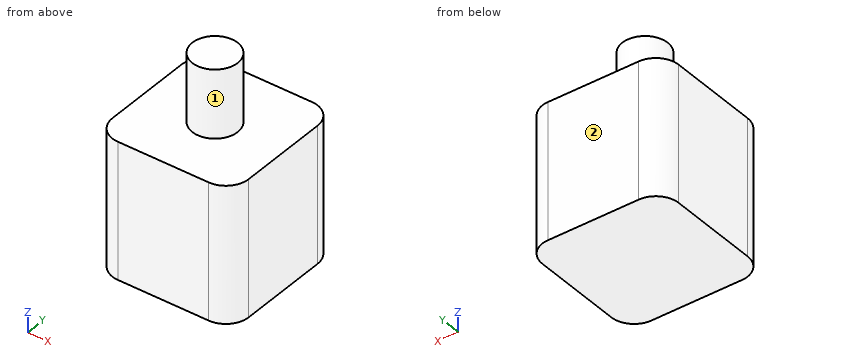
from build123d import *

# Parameters (mm, degrees)
SKETCH1_W           = 60
SKETCH1_H           = 60
BOSS_EXTRUDE1_DEPTH = 30
SKETCH2_R           = 10
BOSS_EXTRUDE2_DEPTH = 30
FILLET1_R           = 10


with BuildPart() as part:
    # Sketch1 → Boss-Extrude1 (new body, symmetric)
    with BuildSketch(Plane.XY):
        Rectangle(SKETCH1_W, SKETCH1_H)
    extrude(amount=BOSS_EXTRUDE1_DEPTH, both=True)

    # Sketch2 → Boss-Extrude2 (add)
    with BuildSketch(Plane.XY.offset(30)):
        Circle(SKETCH2_R)
    extrude(amount=BOSS_EXTRUDE2_DEPTH)

    # Fillet1
    fillet1_edges = [part.edges().sort_by_distance(p)[0] for p in [
        (30, -30, 0),
        (-30, -30, 0),
        (-30, 30, 0),
        (30, 30, 0),
    ]]
    fillet(fillet1_edges, radius=FILLET1_R)


solid = part.part
Work out the finished part from the listing and answer in its coordinate system (mm). Face numbers are marked on the shaded views. A direction names the side the tool comes from. Round coordinates to 2 decimals unless told otherwise and drop trailing zeros. Loops run counter-clockwise (first coordinate to the right, second up) from the corner with the lowest first, then second, coordinate; pieces in that order, holes last. Notation, with made-up numbers: (39.25, 36) - (59.25, 36) arc R13 cw to (59.25, 51) - close; hole circle Ø6 at (-11.75, -3). An arc over 180 degrees is marked (long way). Use one line per item in the form item = value. Start each with the question number.
(1) Find section C-C on z = 45. Determine the outline of the cut face in (x, y).
(2) Which of the six approach directions +Z, -Z, +X, -X, +Y, -Y give full straight-line access (tool end or side, diameter ignored) to the marked faces 1 and 2?
(3) Find section A-A on y = 0. Determine the outline of the cut face in (x, z), and give its area (3 significant figures).
(4) Find section D-D on y = -18. Determine the outline of the cut face in (x, z), and give its area (3 significant figures).
(5) Consider line 1 (Z direction, x = -25, y = -5.5); line 2 (Y direction, x = -22, z = 24.5); line 3 (Y direction, x = 27, z = -12). Determine where each line is inside the solid, lowest interval first.
(6) Flat-ended cylindrical pins translate along their axes: P1, Ø8, axis at y = -3.5, z = 40, coming from the -X side; P2, Ø12, axis at x = -18, y = 4.5, coming from the +Z side. Find the tip coordinate at first contact, or state that the pin passes through.
Answer list:
q1.outline = circle Ø20 at (0, 0)
q2.face_1 = +Z
q2.face_2 = +Z, -Z, +X, -X, +Y
q3.outline = (-30, -30) - (30, -30) - (30, 30) - (10, 30) - (10, 60) - (-10, 60) - (-10, 30) - (-30, 30) - close
q3.area = 4,200 mm^2
q4.outline = (-30, -30) - (30, -30) - (30, 30) - (-30, 30) - close
q4.area = 3,600 mm^2
q5.line_1 = -30 to 30
q5.line_2 = -29.8 to 29.8
q5.line_3 = -27.14 to 27.14
q6.P1 = -10
q6.P2 = 30
